```python
from build123d import *

# Parameters (mm, degrees)
SKETCH1_W           = 150
SKETCH1_H           = 150
BOSS_EXTRUDE1_DEPTH = 50
SKETCH2_W           = 50
SKETCH2_H           = 50
CUT_EXTRUDE1_DEPTH  = 50
CUT_EXTRUDE2_DEPTH  = 50


with BuildPart() as part:
    # Sketch1 → Boss-Extrude1 (new body)
    with BuildSketch(Plane.XY):
        Rectangle(SKETCH1_W, SKETCH1_H)
    extrude(amount=BOSS_EXTRUDE1_DEPTH)

    # Sketch2 → Cut-Extrude1 (cut)
    with BuildSketch(Plane.XY.offset(50)):
        with Locations((-50, 50)):
            Rectangle(SKETCH2_W, SKETCH2_H)
        with Locations((50, 50)):
            Rectangle(SKETCH2_W, SKETCH2_H)
        with Locations((50, -50)):
            Rectangle(SKETCH2_W, SKETCH2_H)
        with Locations((-50, -50)):
            Rectangle(SKETCH2_W, SKETCH2_H)
    extrude(amount=-CUT_EXTRUDE1_DEPTH, mode=Mode.SUBTRACT)

    # Sketch3 → Cut-Extrude2 (cut)
    with BuildSketch(Plane(origin=(0, 25, 0), x_dir=(1, 0, 0), z_dir=(0, 1, 0))):
        Polygon((25, -50), (75, -10), (75, -50), align=None)
        Polygon((-75, -10), (-75, -50), (-25, -50), align=None)
    extrude(amount=-CUT_EXTRUDE2_DEPTH, mode=Mode.SUBTRACT)


solid = part.part
```
Geometry check sheet. Reference: the model listing, model coordinates, mm. A direction names the side the tool comes from. Round coordinates to 2 decimals unless told otherwise and drop trailing zeros. Loops run counter-clockwise (first coordinate to the right, second up) from the corner with the lowest first, then second, coordinate; pieces in that order, holes last. Notation, with made-up numbers: (59, 34) -> (111, 34) arc R19 cw to (111, 38) -> close; hole circle Ø5 at (-16.5, -32.75). An arc over 180 degrees is marked (long way). Use a Markdown table: item, result.
(1) Sectioned sample at A-A (y = -12.5). Enter the section's corners in (x, z), then the cut area to 3 significant figures.
Calculated:
| item | result |
|---|---|
| outline | (-75, 0) -> (75, 0) -> (75, 10) -> (25, 50) -> (-25, 50) -> (-75, 10) -> close |
| area | 5,500 mm² |
(2) Go/stop test with flat-tipped pins: P1, Ø5, axis at x = -43, z = 17, coming from the -Y side; P2, Ø6, axis at y = -14, z = 39, coming from the -X side; P3, Ø25, axis at y = 46, z = 22, coming from the +X side. Record where each tip stops, or that it passes through.
Calculated:
| item | result |
|---|---|
| P1 | y = -25 |
| P2 | x = -42.5 |
| P3 | x = 25 |
(3) Set-up check for faces 1 (the flat face through (-25, -50, 25)), 2 (the flat face through (44, 25, 20)), 3 (the flat face through (44, -25, 20)): record each of +Z, -Z, +X, -X, +Y, -Y from which the full face is reachable in a straight line by a thin tool's end or side.
Calculated:
| item | result |
|---|---|
| face 1 | +Z, -Z, -X, -Y |
| face 2 | +Z, -Z, +X, +Y |
| face 3 | +Z, -Z, +X, -Y |
(4) Sectioned sample at C-C (x = -61). Enter the section's corners in (y, z).
Calculated:
| item | result |
|---|---|
| outline | (-25, 0) -> (25, 0) -> (25, 21.2) -> (-25, 21.2) -> close |
(5) Sectioned sample at D-D (z = 25.5). Enter the section's corners in (x, y) (3 decimals), then the cut area to 3 significant figures.
Calculated:
| item | result |
|---|---|
| outline | (-55.625, -25) -> (-25, -25) -> (-25, -75) -> (25, -75) -> (25, -25) -> (55.625, -25) -> (55.625, 25) -> (25, 25) -> (25, 75) -> (-25, 75) -> (-25, 25) -> (-55.625, 25) -> close |
| area | 10,600 mm² |
(6) Scan lines: probe 1 along Y at (x, z) = (28.5, 47); probe 2 along X at (y, z) = (-14, 43). Record each from-to range of solid material in increasing order.
Calculated:
| item | result |
|---|---|
| probe 1 | -25 to 25 |
| probe 2 | -33.75 to 33.75 |
(7) Sectioned sample at B-B (z = 35). Enter the section's corners in (x, y), then the cut area to 4 significant figures.
Calculated:
| item | result |
|---|---|
| outline | (-43.75, -25) -> (-25, -25) -> (-25, -75) -> (25, -75) -> (25, -25) -> (43.75, -25) -> (43.75, 25) -> (25, 25) -> (25, 75) -> (-25, 75) -> (-25, 25) -> (-43.75, 25) -> close |
| area | 9,375 mm² |
